The figure shows three views and two pictorial views of one solid part (mm, origin at its lowest corner). Answer the questions. A direction names the side the tool comes from. Coordinates: 2 decimals unless noted, no trailing zeros. Loops run counter-clockwise (first coordinate to the right, second up) from the corner with the lowest first, then second, coordinate; pieces in that order, holes last. Notation, with made-up numbers: M 20,-36 L 54,-36 A19 cw 54,-29 Z; hole C 15.25,11 d9. An arc over 180 degrees is marked long. One line per item, written item: value. Start each with the question number.
1. Consider probe 1 along X at (y, z) = (8.5, 0.55); probe 2 along Y at (x, z) = (6, 1.4); probe 3 along X at (y, z) = (14.25, 1.35). Determine where each line is inside the solid, lowest interval first.
2. The part is cut by section A-A (y = 8.25). Write down the section's boundary in (x, z).
3. Determine the mould class of the marked faces 1, 2, 3 and 4 for opening direction Y: +Y half, -Y half, draft (parallel to the pull), parting line (faces both ways), or undercut.
4. For the marked faces 5, 6 and 7, determine the directions among +Z, -Z, +X, -X, +Y, -Y from which every point of the face is accessible in a straight line to the end or side of a thin tool.
5. The part is cut by section D-D (x = 6). Write down the section's boundary in (y, z).
6. The part is cut by section B-B (x = 2.5). Write down the section's boundary in (y, z) (1 decimal).
7. Flat-ended cylindrical pins translate along their axes: pin 1 (1.5 mm diameter, centred on y = 18, z = 2.5, fed in from -X); pin 2 (3 mm diameter, centred on x = 3.5, z = 3, fed in from +Y). Find the tip coordinate at first contact, or state that the pin passes through.
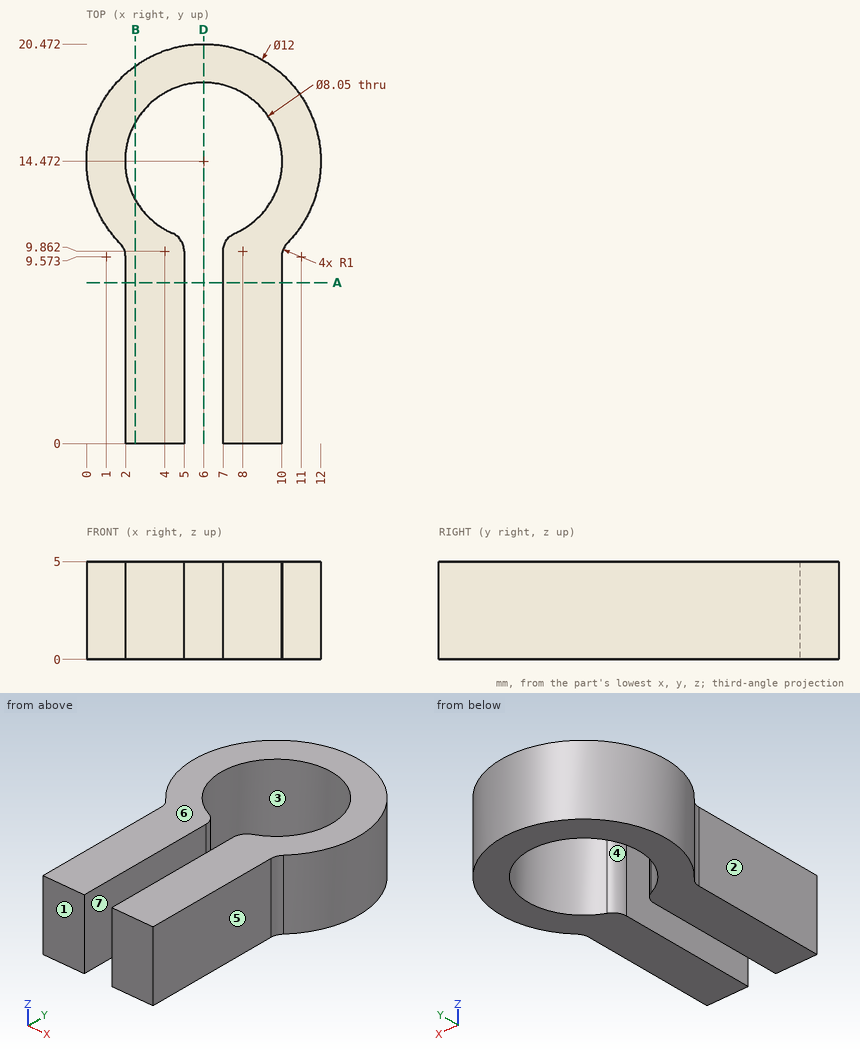
Answer block:
1. probe 1: x = 2 to 5, 7 to 10
1. probe 2: y = 18.5 to 20.47
1. probe 3: x = 0 to 1.98, 10.02 to 12
2. outline: M 2,0 L 5,0 L 5,5 L 2,5 Z; M 7,0 L 10,0 L 10,5 L 7,5 Z
3. face 1: -Y half
3. face 2: draft
3. face 3: undercut
3. face 4: undercut
4. face 5: +Z, -Z, +X, -Y
4. face 6: +Z, +X, -X, +Y, -Y
4. face 7: +Z, -Z, -Y
5. outline: M 18.5,0 L 20.47,0 L 20.47,5 L 18.5,5 Z
6. outline: M 0,0 L 12.5,0 L 12.5,5 L 0,5 Z; M 16.5,0 L 19.3,0 L 19.3,5 L 16.5,5 Z
7. pin 1: stops at x = 0.68
7. pin 2: stops at y = 20.39
